Input: part model. Units: mm. Frame: model coordinates. Face numbers are marked on the shaded views. Round coordinates to 2 decimals unless told otherwise and drop trailing zeros. Write each loop counter-clockwise with the first axis right and the second up, starting at its lowest first coordinate (ties: lowest second). Pieces come first, ordered by that corner, then holes. Notation, with made-up numbers: (-31.5, -20.75) -> (-10.5, -20.75) arc R14 cw to (-10.5, -5.75) -> close; hole circle Ø5 at (89, 23). An arc over 180 degrees is marked (long way). Use CSV: the item, a comma, the result in double quotes.
Autodesk Inventor part; units mm, degrees
ref_plane "YZ Plane" through (0, 0, 0) normal (1, 0, 0) x (0, 1, 0)
ref_plane "XZ Plane" through (0, 0, 0) normal (0, 1, 0) x (-1, 0, 0)
ref_plane "XY Plane" through (0, 0, 0) normal (0, 0, 1) x (1, 0, 0)
sketch "Sketch1" plane through (0, 0, 0) normal (1, 0, 0) x (0, 1, 0)
  line L0 (0, 0) -> (0, -50.8)
  line L1 (0, -50.8) -> (412.242, -50.8)
  line L2 (412.242, -50.8) -> (412.242, 0)
  line L3 (412.242, 0) -> (0, 0)
  line L4 (412.242, -25.4) -> (0, -25.4) construction
  circle A0 centre (82.042, -25.4) radius 11.1125
  circle A1 centre (393.192, -25.4) radius 11.1125
  line L5 (0, -13.97) -> (412.242, -13.97) construction
  line L6 (132.842, -13.97) -> (132.842, -36.83) construction
  line L7 (342.392, -13.97) -> (342.392, -36.83) construction
  circle A2 centre (132.842, -36.83) radius 11.1125
  circle A3 centre (342.392, -36.83) radius 11.1125
  line L8 (132.842, -36.83) -> (342.392, -36.83) construction
  line L9 (160.6042, -15.875) -> (109.8042, -15.875) construction
  circle A4 centre (135.2042, -15.875) radius 9.525
  circle A5 centre (160.6042, -15.875) radius 2.0193
  circle A6 centre (109.8042, -15.875) radius 2.0193
  circle A7 centre (374.142, -9.525) radius 1.5875
  circle A8 centre (374.142, -41.275) radius 1.5875
  circle A9 centre (12.7, -25.4) radius 3.175
  circle A10 centre (28.575, -25.4) radius 3.175
  line L10 (374.142, -41.275) -> (374.142, -9.525) construction
  line L11 (316.992, -12.7) -> (297.942, -12.7) construction
  line L12 (316.992, 0) -> (316.992, -50.8) construction
  circle A11 centre (316.992, -12.7) radius 1.5875
  circle A12 centre (297.942, -12.7) radius 1.5875
  circle A13 centre (316.992, -31.75) radius 1.5875
  point P0 (374.142, -25.4)
  dimension "d0" = 50.8
  dimension "d3" = 22.225
  dimension "d4" = 311.15
  dimension "d5" = 19.05
  dimension "d12" = 82.042
  dimension "d18" = 11.43
  dimension "d19" = 50.8
  dimension "d20" = 50.8
  dimension "d29" = 15.875
  dimension "d30" = 50.8
  dimension "d31" = 53.1622
  dimension "d35" = 4.0386
  dimension "d36" = 19.05
  dimension "d37" = 22.225
  dimension "d38" = 12.7
  dimension "d39" = 15.875
  dimension "d40" = 6.35
  dimension "d41" = 31.75
  dimension "d42" = 19.05
  dimension "d43" = 3.175
  dimension "d44" = 19.05
  dimension "d45" = 19.05
  dimension "d47" = 6.35
  dimension "d48" = 234.95
extrude "Extrusion1" add sketch "Sketch1" along normal blind 3.175
sketch "Sketch2" plane through (0, 0, 0) normal (-1, 0, 0) x (0, 0, 1)
  line L0 (0, 412.242) -> (0, 0)
  line L1 (-50.8, 412.242) -> (0, 412.242) construction
  line L2 (0, 0) -> (-3.175, 0)
  line L3 (-3.175, 0) -> (-3.175, 412.242)
  line L4 (-3.175, 412.242) -> (0, 412.242)
  line L5 (0, 412.242) -> (0, 0)
  line L6 (-50.8, 0) -> (-50.8, 412.242)
  line L7 (-50.8, 0) -> (-47.625, 0)
  line L8 (-47.625, 0) -> (-47.625, 412.242)
  line L9 (-47.625, 412.242) -> (-50.8, 412.242)
  line L10 (-50.8, 412.242) -> (-50.8, 0)
  dimension "d13" = 3.175
  dimension "d14" = 3.175
extrude "Extrusion2" add sketch "Sketch2" along normal blind 9.525
fillet "Fillet2" radius 19.05 2 edges at (-3.175, 412.242, 0) (-3.175, 412.242, -50.8)
equation "\"d20\" = d19"
equation "\"d29\" = d23"
equation "\"d45\" = d44"
equation "\"d14\" = d13"
properties part number "Front C Left"
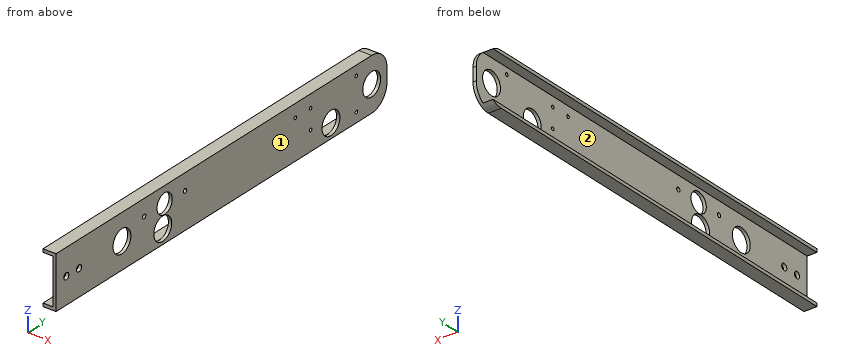
Item 1: Section query A-A on x = -2.75. Return the cut outline in (y, z) (3 decimals).
Worked answers:
outline,"(0, -50.8) -> (393.192, -50.8) arc R19.05 ccw to (403.722, -47.625) -> (0, -47.625) -> close; (0, -3.175) -> (403.722, -3.175) arc R19.05 ccw to (393.192, 0) -> (0, 0) -> close"
Item 2: Line query: line 1 (Z direction, x = -3.5, y = 354) (3 decimals); line 2 (Y direction, x = 2, z = -34); line 3 (Y direction, x = 1.6, z = -36.83). Output: solid intervals per line, ascending.
Worked answers:
line 1,"z = -50.8 to -47.625, -3.175 to 0"
line 2,"y = 0 to 75, 89.08 to 122.1, 143.59 to 331.65, 353.14 to 386.15, 400.23 to 412.11"
line 3,"y = 0 to 121.73, 143.95 to 331.28, 353.5 to 411.55"
Item 3: Pull-direction query (Z, two-part tool) for the marked faces 1 and 2; classes: +Z half, -Z half, draft (parallel to the pull), parting line (faces both ways), or undercut.
Worked answers:
face 1,"draft"
face 2,"undercut"
Item 4: First-contact query: pin 1 Ø3.5 at (y, z) = (374.142, -9.525) entering from -X; pin 2 Ø1.5 at (x, z) = (1, -14) entering from +Y. Flat tips, straight axial feed; report the tip coordinate or a pass-through.
Worked answers:
pin 1,"stops at x = 0"
pin 2,"stops at y = 411.75"
Item 5: Section query B-B on y = 101.5. Return the cut outline in (x, z) (3 decimals).
Worked answers:
outline,"(-9.525, -50.8) -> (3.175, -50.8) -> (3.175, 0) -> (-9.525, 0) -> (-9.525, -3.175) -> (0, -3.175) -> (0, -47.625) -> (-9.525, -47.625) -> close"
